Here's how the part is built. I have some questions about the finished solid (model axes, mm). A direction names the side the tool comes from. Give positions to 0.01 mm unless a question says otherwise; leave off trailing zeros. Write each loop counter-clockwise with the first axis right and the second up, starting at its lowest first coordinate (ties: lowest second). Pieces come first, ordered by that corner, then holes. Notation, with made-up numbers: (-8, 31) -> (27, 31) arc R18 cw to (27, 35) -> close; hole circle Ø9 at (50, -4.5). An arc over 180 degrees is marked (long way). Use one line per item in the form item = value.
```python
from build123d import *

# Parameters (mm, degrees)
BOSS_EXTRUDE1_DEPTH = 76.2
CUT_EXTRUDE1_DEPTH  = 10
SKETCH4_R           = 3.5
CUT_EXTRUDE2_DEPTH  = 10


with BuildPart() as part:
    # Sketch2 → Boss-Extrude1 (new body, symmetric)
    with BuildSketch(Plane.XY):
        with BuildLine():
            Line((-38.1, 0), (38.1, 0))
            Line((38.1, 0), (38.1, 76.2))
            Line((38.1, 76.2), (34.925, 76.2))
            ThreePointArc((34.925, 76.2), (32.67993597, 75.27006403), (31.75, 73.025))
            Line((31.75, 73.025), (31.75, 9.525))
            ThreePointArc((31.75, 9.525), (30.82006403, 7.27993597), (28.575, 6.35))
            Line((28.575, 6.35), (-34.925, 6.35))
            ThreePointArc((-34.925, 6.35), (-37.17006403, 5.42006403), (-38.1, 3.175))
            Line((-38.1, 3.175), (-38.1, 0))
        make_face()
    extrude(amount=BOSS_EXTRUDE1_DEPTH, both=True)

    # Sketch3 → Cut-Extrude1 (cut)
    with BuildSketch(Plane(origin=(38.1, 0, 0), x_dir=(0, 0, -1), z_dir=(1, 0, 0))):
        with BuildLine():
            Line((-28.25, 65.4), (-28.25, 14.6))
            ThreePointArc((-28.25, 14.6), (-31.75, 11.1), (-35.25, 14.6))
            Line((-35.25, 14.6), (-35.25, 65.4))
            ThreePointArc((-35.25, 65.4), (-31.75, 68.9), (-28.25, 65.4))
        make_face()
        with BuildLine():
            Line((28.25, 65.4), (28.25, 14.6))
            ThreePointArc((28.25, 14.6), (31.75, 11.1), (35.25, 14.6))
            Line((35.25, 14.6), (35.25, 65.4))
            ThreePointArc((35.25, 65.4), (31.75, 68.9), (28.25, 65.4))
        make_face()
        with BuildLine():
            Line((3.5, 65.4), (3.5, 14.6))
            ThreePointArc((3.5, 14.6), (0, 11.1), (-3.5, 14.6))
            Line((-3.5, 14.6), (-3.5, 65.4))
            ThreePointArc((-3.5, 65.4), (0, 68.9), (3.5, 65.4))
        make_face()
    extrude(amount=-CUT_EXTRUDE1_DEPTH, mode=Mode.SUBTRACT)

    # Sketch4 → Cut-Extrude2 (cut)
    with BuildSketch(Plane.XZ):
        with Locations((-12.35, 25.4)):
            Circle(SKETCH4_R)
        with Locations((-12.35, -25.4)):
            Circle(SKETCH4_R)
        with Locations((-12.35, 0)):
            Circle(SKETCH4_R)
    extrude(amount=-CUT_EXTRUDE2_DEPTH, mode=Mode.SUBTRACT)


solid = part.part
```
Q1. I want a section at D-D, the plane z = -48. Write out the boundary of the cut face in (x, y) (3 decimals).
Result set:
outline = (-38.1, 0) -> (38.1, 0) -> (38.1, 76.2) -> (34.925, 76.2) arc R3.175 ccw to (31.75, 73.025) -> (31.75, 9.525) arc R3.175 cw to (28.575, 6.35) -> (-34.925, 6.35) arc R3.175 ccw to (-38.1, 3.175) -> close
Q2. I want a section at C-C, the plane y = 45. Write out the boundary of the cut face in (x, z), and give its area (3 significant figures).
Result set:
outline = (31.75, -76.2) -> (38.1, -76.2) -> (38.1, -35.25) -> (31.75, -35.25) -> close; (31.75, -28.25) -> (38.1, -28.25) -> (38.1, -3.5) -> (31.75, -3.5) -> close; (31.75, 3.5) -> (38.1, 3.5) -> (38.1, 28.25) -> (31.75, 28.25) -> close; (31.75, 35.25) -> (38.1, 35.25) -> (38.1, 76.2) -> (31.75, 76.2) -> close
area = 834 mm2
Q3. Will these pins go through, and if not, where does the flat tip stop? pin 1 Ø2 at (y, z) = (50.5, 25.5) entering from -X; pin 2 Ø1 at (x, z) = (18, -38) entering from +Y.
Result set:
pin_1 = 31.75
pin_2 = 6.35
Q4. I want a section at A-A, the plane z = 31.75. Write out the boundary of the cut face in (x, y) (3 decimals), and give its area (3 significant figures).
Result set:
outline = (-38.1, 0) -> (38.1, 0) -> (38.1, 11.1) -> (31.75, 11.1) -> (31.75, 9.525) arc R3.175 cw to (28.575, 6.35) -> (-34.925, 6.35) arc R3.175 ccw to (-38.1, 3.175) -> close; (31.75, 68.9) -> (38.1, 68.9) -> (38.1, 76.2) -> (34.925, 76.2) arc R3.175 ccw to (31.75, 73.025) -> close
area = 558 mm2
Q5. If I drill on line 1 along Z through (x, y) = (-12.35, 3.5); line 2 along X through (y, z) = (58.5, -41); line 3 along Y through (x, z) = (2, -24), over which ranges is the centre line in solid material (lowest first)? Write a range as from..to.
Result set:
line_1 = -76.2..-28.9, -21.9..-3.5, 3.5..21.9, 28.9..76.2
line_2 = 31.75..38.1
line_3 = 0..6.35
Q6. Which directions (+Z, -Z, +X, -X, +Y, -Y) give clear straight access to the entire face, cutting with the end or side of a thin tool? Please do faces 1 (the face through (-1, 0, 1)), 2 (the face through (35, 40, 35.25)), 3 (the face through (-3, 6.35, 1)).
Result set:
face_1 = +Z, -Z, +X, -X, -Y
face_2 = +X, -X
face_3 = +Z, -Z, -X, +Y
Q7. If we mould it in two halves opening along Y, with no side actions, what happens to faces 4 (the face through (-9.1, 3.1, -1.3)), 5 (the face through (35, 40, -3.5)), 6 (the face through (35, 40, 3.5)), 7 (the face through (-37.15, 5.44, 1.07))? For each: +Y half, -Y half, draft (parallel to the pull), parting line (faces both ways), or undercut.
Result set:
face_4 = draft
face_5 = undercut
face_6 = undercut
face_7 = +Y half
Q8. I want a section at B-B, the plane z = 0. Write out the boundary of the cut face in (x, y) (3 decimals), and give its area (3 significant figures).
Result set:
outline = (-38.1, 0) -> (-15.85, 0) -> (-15.85, 6.35) -> (-34.925, 6.35) arc R3.175 ccw to (-38.1, 3.175) -> close; (-8.85, 0) -> (38.1, 0) -> (38.1, 11.1) -> (31.75, 11.1) -> (31.75, 9.525) arc R3.175 cw to (28.575, 6.35) -> (-8.85, 6.35) -> close; (31.75, 68.9) -> (38.1, 68.9) -> (38.1, 76.2) -> (34.925, 76.2) arc R3.175 ccw to (31.75, 73.025) -> close
area = 514 mm2
